Source: CAD feature listing. Evaluate the final solid. Frame: model axes, mm. A direction names the side the tool comes from. Give positions to 0.01 mm unless a question says otherwise; leave off trailing zeros. Order: outer loops, then holes, each group sorted by start corner. A loop starts at its lowest first (then second) coordinate and runs counter-clockwise, first axis right, second up.
Solid Edge part; units mm, degrees
sketch "Sketch1" plane through (0, 0, 0) normal (0, 0, 1) x (1, 0, 0)
  line L0 (-23, -6) -> (23, -6)
  arc A0 (23, 6) -> (23, -6) centre (23, 0) cw
  line L1 (23, 6) -> (-23, 6)
  arc A1 (-23, 6) -> (-23, -6) centre (-23, 0) ccw
  arc A2 (-28.8095, 1.5) -> (-28.8095, -1.5) centre (-23, 0) ccw
  line L2 (-28.8095, -1.5) -> (-25, -1.5)
  line L3 (-25, -1.5) -> (-25, 1.5)
  line L4 (-25, 1.5) -> (-28.8095, 1.5)
extrude "Protrusion1" add sketch "Sketch1" against normal blind 2
fillet "Round_1" radius 2 4 edges at (0, -6, 0) (29, 0, 0) (0, 6, 0) (-29, 0, 0)
sketch "Sketch2" plane through (0, 0, 0) normal (0, 0, 1) x (1, 0, 0)
  line L0 (-28.8095, -1.5) -> (-25, -1.5)
  line L1 (-25, -1.5) -> (-25, 1.5)
  line L2 (-25, 1.5) -> (-28.8095, 1.5)
  arc A0 (-28.8095, 1.5) -> (-28.8095, -1.5) centre (-23, 0) ccw
extrude "ExtrudedCutout_1" cut sketch "Sketch2" against normal blind 2
sketch "Sketch3" plane through (0.0953, 0, -2) normal (0, 0, -1) x (-1, 0, 0)
  line L0 (-19.9047, -1.5) -> (25.0953, -1.5)
  line L1 (25.0953, -1.5) -> (25.0953, 1.5)
  line L2 (25.0953, 1.5) -> (-19.9047, 1.5)
  line L3 (-19.9047, 1.5) -> (-19.9047, -1.5)
extrude "ExtrudedCutout_2" cut sketch "Sketch3" against normal blind 1.25
sketch "Sketch4" plane through (0.0953, 0, -2) normal (0, 0, -1) x (-1, 0, 0)
  circle A0 centre (23.0953, -3) radius 1
extrude "ExtrudedCutout_3" cut sketch "Sketch4" against normal blind 1.75
sketch "Sketch5" plane through (0.0953, 0, -2) normal (0, 0, -1) x (-1, 0, 0)
  circle A0 centre (23.0953, 3) radius 1
extrude "ExtrudedCutout_4" cut sketch "Sketch5" against normal blind 1.75
sketch "Sketch6" plane through (0.0953, 0, -2) normal (0, 0, -1) x (-1, 0, 0)
  circle A0 centre (-22.9047, -3) radius 1
extrude "ExtrudedCutout_6" cut sketch "Sketch6" against normal blind 1.75
sketch "Sketch7" plane through (0.0953, 0, -2) normal (0, 0, -1) x (-1, 0, 0)
  circle A0 centre (-22.9047, 3) radius 1
extrude "ExtrudedCutout_7" cut sketch "Sketch7" against normal blind 1.75
sketch "Sketch8" plane through (0.0953, 0, -2) normal (0, 0, -1) x (-1, 0, 0)
  circle A0 centre (-25.9047, 0) radius 1.5
extrude "ExtrudedCutout_8" cut sketch "Sketch8" against normal blind 1
sketch "Sketch9" plane through (-25, 0, -0.375) normal (-1, 0, 0) x (0, 0, 1)
  line L0 (-0.375, 1.5) -> (-0.375, -1.5)
  line L1 (-0.375, -1.5) -> (-0.175, -1.5)
  line L2 (-0.175, -1.5) -> (-0.175, 1.5)
  line L3 (-0.175, 1.5) -> (-0.375, 1.5)
extrude "ExtrudedCutout_9" cut sketch "Sketch9" against normal blind 45
1) First-contact query: pin 1 Ø1.5 at (x, y) = (26.5, 0) entering from -Z; pin 2 Ø1 at (x, y) = (-23.5, -2.5) entering from -Z; pin 3 Ø1 at (x, z) = (-27, -0.5) entering from -Y; pin 4 Ø1.5 at (x, y) = (6.5, 0.5) entering from -Z. Flat tips, straight axial feed; report the tip coordinate or a pass-through.
Checks:
pin 1: stops at z = -1
pin 2: stops at z = -2
pin 3: stops at y = -4.3
pin 4: stops at z = -0.55
2) Pull-direction query (X, two-part tool) for faces 3 (the face through (-3, 0, -0.55)), 4 (the face through (27.5, 0.07, -1.51)), 5 (the face through (20, 0, -1)); classes: +X half, -X half, draft (parallel to the pull), parting line (faces both ways), or undercut.
Checks:
face 3: draft
face 4: undercut
face 5: -X half
3) Section query A-A on x = -8. Output: boundary loops of the cut face in (y, z), and give its area (3 significant figures).
Checks:
outline: (-6, -2) - (-1.5, -2) - (-1.5, -0.55) - (1.5, -0.55) - (1.5, -2) - (6, -2) arc R2 ccw to (4, 0) - (-4, 0) arc R2 ccw to start
area: 17.9 mm2
4) Section query B-B on y = 0. Output: boundary loops of the cut face in (x, z).
Checks:
outline: (-25, -0.55) - (20, -0.55) - (20, -2) - (24.5, -2) - (24.5, -1) - (27.5, -1) - (27.5, -2) - (29, -2) arc R2 ccw to (27, 0) - (-25, 0) - close
5) Ray query, L1, parallel to X at y = -3.5, z = -1.1; L2, parallel to Y at x = 3, z = -1.8; L3, parallel to Y at x = -23, z = -1.25. Return the intervals inside material, ascending.
Checks:
L1: x = -27.61 to -23.87, -22.13 to 22.13, 23.87 to 27.61
L2: y = -5.99 to -1.5, 1.5 to 5.99
L3: y = -5.85 to -4, -2 to -1.5, 1.5 to 2, 4 to 5.85
6) Reachability of faces 1 (the face through (-0.32, -5.43, -0.6)), 2 (the face through (26, 0, -1)) from +Z, -Z, +X, -X, +Y, -Y: full face, straight path, thin tool, end or side. Return the list, or none.
Checks:
face 1: +Z, +X, -X, -Y
face 2: -Z
